Check sheet for the drawn part. Datum: minimum x, y, z corner. Units: mm. Round coordinates to 2 decimals unless told otherwise and drop trailing zeros. Write each loop counter-clockwise with the first axis right and the second up, starting at its lowest first coordinate (ties: lowest second). Pieces come first, ordered by that corner, then holes.
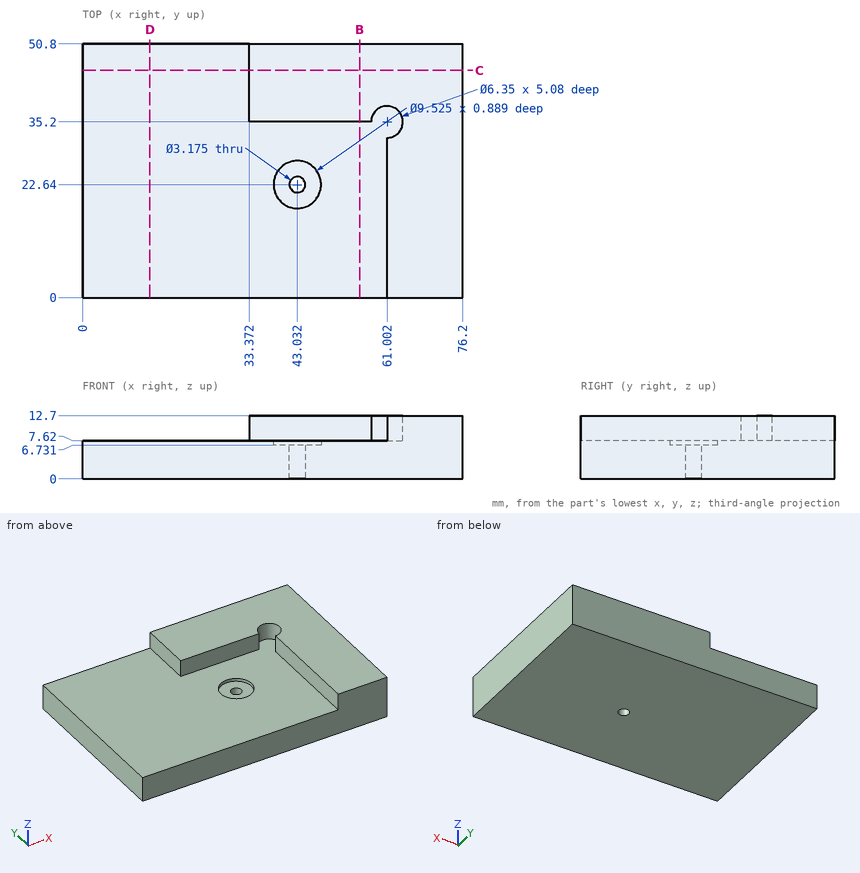
Q1. Depth check by flat-ended pin: P1, Ø8, axis at x = 43, y = 13, coming from the +Z side; P2, Ø5, axis at x = 61, y = 35.2, coming from the -Z side; P3, Ø5.5, axis at y = 44.5, z = 11.5, coming from the -X side; P4, Ø1.9, axis at x = 43.03, y = 22.64, coming from the +Z side. Enter the tip coordinate at first touch or a pass-through.
Recorded:
P1: stops at z = 7.62
P2: stops at z = 0
P3: stops at x = 33.37
P4: passes through
Q2. Sectioned sample at C-C (y = 45.5). Enter the section's corners in (x, z).
Recorded:
outline: (0, 0) - (76.2, 0) - (76.2, 12.7) - (33.37, 12.7) - (33.37, 7.62) - (0, 7.62) - close
Q3. Material ranges on line 1 along X through (y, z) = (41, 8.5); line 2 along Z through (x, y) = (25, 44.5); line 3 along Y through (x, z) = (36, 12.25), recorded low to high.
Recorded:
line 1: x = 33.37 to 76.2
line 2: z = 0 to 7.62
line 3: y = 35.2 to 50.8
Q4. Sectioned sample at B-B (x = 55.5). Enter the section's corners in (y, z), plus the area to 3 significant figures.
Recorded:
outline: (0, 0) - (50.8, 0) - (50.8, 12.7) - (35.2, 12.7) - (35.2, 7.62) - (0, 7.62) - close
area: 466 mm2
Q5. Sectioned sample at D-D (x = 13.5). Enter the section's corners in (y, z), plus the area to 3 significant figures.
Recorded:
outline: (0, 0) - (50.8, 0) - (50.8, 7.62) - (0, 7.62) - close
area: 387 mm2
